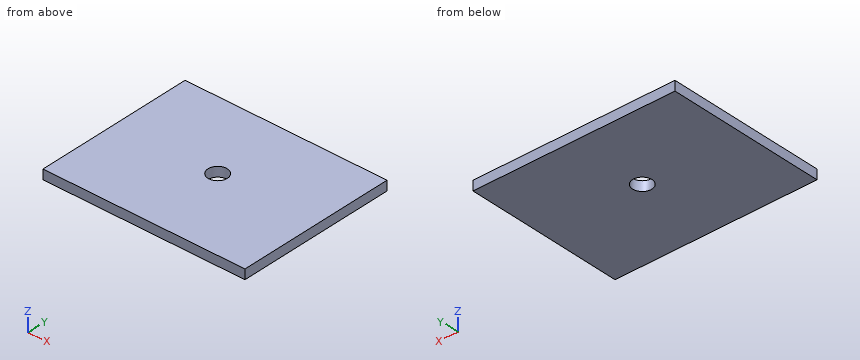
from build123d import *

# Parameters (mm, degrees)
CYLINDER_R     = 2
CYLINDER_DEPTH = 10
SKETCH_W       = 41.771851
SKETCH_H       = 33.013145
EXTRUDE_DEPTH  = 2


with BuildPart() as cilindro:
    # Cylinder → Cylinder (new body)
    with BuildSketch(Plane(origin=(21, 17, -4), x_dir=(1, 0, 0), z_dir=(0, 0, 1))):
        Circle(CYLINDER_R)
    extrude(amount=CYLINDER_DEPTH)


with BuildPart() as cut:
    # Sketch → Extrude (new body)
    with BuildSketch(Plane.XY):
        with Locations((20.885925, 16.506573)):
            Rectangle(SKETCH_W, SKETCH_H)
    extrude(amount=EXTRUDE_DEPTH)

    # Cut: cut Cilindro
    add(cilindro.part, mode=Mode.SUBTRACT)


solid = cut.part
Part model, mm, in its own coordinate system. Coordinates: 2 decimals unless noted, no trailing zeros. Loops run counter-clockwise (first coordinate to the right, second up) from the corner with the lowest first, then second, coordinate; pieces in that order, holes last. Notation, with made-up numbers: (0.5, -4.5) -> (24.5, -4.5) arc R22 cw to (24.5, 27.5) -> close; hole circle Ø8 at (-8, 84). An arc over 180 degrees is marked (long way). Use a Markdown table: item, result. Add a question column.
Item 1: Band-saw the part on A-A on x = 21. Write the cut outline in (y, z).
Item 2: Flat gauge pin, fed straight in: P1, Ø4.5, axis at x = 21, y = 17, coming from the +Z side. Where does the tip first touch, or does it go through?
Item 3: Probe probe 1 along X at (y, z) = (17, 0.9); probe 2 along Y at (x, z) = (21, 1.05); probe 3 along Y at (x, z) = (21.5, 0.2). List the from-to ranges inside material, lowest first.
Item 4: Band-saw the part on B-B on y = 17. Write the cut outline in (x, z), plus the area to 3 significant figures.
Geometry says:
| question | item | result |
|---|---|---|
| 1 | outline | (0, 0) -> (15, 0) -> (15, 2) -> (0, 2) -> close; (19, 0) -> (33.01, 0) -> (33.01, 2) -> (19, 2) -> close |
| 2 | P1 | z = 2 |
| 3 | probe 1 | 0 to 19, 23 to 41.77 |
| 3 | probe 2 | 0 to 15, 19 to 33.01 |
| 3 | probe 3 | 0 to 15.06, 18.94 to 33.01 |
| 4 | outline | (0, 0) -> (19, 0) -> (19, 2) -> (0, 2) -> close; (23, 0) -> (41.77, 0) -> (41.77, 2) -> (23, 2) -> close |
| 4 | area | 75.5 mm² |
